Here's how the part is built. I have some questions about the finished solid (model axes, mm). A direction names the side the tool comes from. Round coordinates to 2 decimals unless told otherwise and drop trailing zeros. Write each loop counter-clockwise with the first axis right and the second up, starting at its lowest first coordinate (ties: lowest second). Pieces come first, ordered by that corner, then holes. Notation, with made-up numbers: (38.5, 38.5) -> (63.5, 38.5) arc R18 cw to (63.5, 48.5) -> close; hole circle Ø8 at (2.25, 36). An arc over 180 degrees is marked (long way). Answer in a Markdown table with one row per item.
from build123d import *

# Parameters (mm, degrees)
F0_R      = 50
F1_DEPTH  = 198
F1_TAPER  = -5
F1_FACE_R = 67.3227553781
F2_DEPTH  = 103
F2_TAPER  = 5
F3_DEPTH  = 25
F3_FACE_R = 58.311423035
F4_DEPTH  = 25
F4_TAPER  = -20
F5_R      = 45
F6_DEPTH  = 304


with BuildPart() as f1:
    # F0 (on Top) → F1 (new body)
    with BuildSketch(Plane.XY):
        Circle(F0_R)
    extrude(amount=F1_DEPTH, taper=F1_TAPER)

    # F1_face (on face) → F2 (join)
    with BuildSketch(Plane.XY.offset(198)):
        Circle(F1_FACE_R)
    extrude(amount=F2_DEPTH, taper=F2_TAPER)

    # F3 (add): a face of the model
    f3_faces = [f1.faces().sort_by_distance(p)[0] for p in [
        (0, 0, 301),
    ]]
    extrude(f3_faces, amount=F3_DEPTH)

    # F3_face (on face) → F4 (join)
    with BuildSketch(Plane.XY.offset(326)):
        Circle(F3_FACE_R)
    extrude(amount=F4_DEPTH, taper=F4_TAPER)

    # F5 (on face) → F6 (cut)
    with BuildSketch(Plane.XY.offset(351)):
        Circle(F5_R)
    extrude(amount=-F6_DEPTH, mode=Mode.SUBTRACT)


solid = f1.part
1) We'd pull the mould along Z, two halves only. Please class faces 4 (the face through (54, 22, 313)), 5 (the face through (-46.648, -35.768, 100.386)), 6 (the face through (14, -44, 351)): +Z half, -Z half, draft (parallel to the pull), parting line (faces both ways), or undercut.
Response:
| item | result |
|---|---|
| face 4 | undercut |
| face 5 | -Z half |
| face 6 | +Z half |
2) Which directions (+Z, -Z, +X, -X, +Y, -Y) give clear straight access to the entire face, cutting with the end or side of a thin tool? Please do faces 1 (the face through (-12.76, -57.48, 327.56)), 2 (the face through (-1, 1, 0)), 3 (the face through (-1, 1, 47)).
Response:
| item | result |
|---|---|
| face 1 | none |
| face 2 | -Z, +X, -X, +Y, -Y |
| face 3 | +Z |
3) I want a section at B-B, the plane z = 321.5. List the corners of the cut face in (x, y) for me.
Response:
| item | result |
|---|---|
| outline | circle Ø116.62 at (0, 0); hole circle Ø90 at (0, 0) |
4) For pin 1 (2 mm diameter, centred on y = -26.5, z = 179.5, fed in from +X); pin 2 (12 mm diameter, centred on x = -15, y = 23.5, fed in from +Z); pin 3 (8 mm diameter, centred on y = -26.5, z = 117, fed in from +X); pin 4 (6 mm diameter, centred on x = -39.5, y = -35, fed in from -Z), each with a flat end and sliding along its axis, tell me the tip position at first contact or that it passes through.
Response:
| item | result |
|---|---|
| pin 1 | stops at x = 60.56 |
| pin 2 | stops at z = 47 |
| pin 3 | stops at x = 55.92 |
| pin 4 | stops at z = 0 |
5) I want a section at C-C, the plane z = 231.5. List the corners of the cut face in (x, y) for me.
Response:
| item | result |
|---|---|
| outline | circle Ø128.78 at (0, 0); hole circle Ø90 at (0, 0) |
6) I want a section at A-A, the plane x = 0. List the corners of the cut face in (y, z) for me, and give its area (3 significant figures).
Response:
| item | result |
|---|---|
| outline | (-67.41, 351) -> (-58.31, 326) -> (-58.31, 301) -> (-67.32, 198) -> (-50, 0) -> (50, 0) -> (67.32, 198) -> (58.31, 301) -> (58.31, 326) -> (67.41, 351) -> (45, 351) -> (45, 47) -> (-45, 47) -> (-45, 351) -> close |
| area | 14,900 mm^2 |
7) I need wall thicknesses on line 1 (Z direction, x = 12, y = 34.5); line 2 (Y direction, x = 0, z = 287); line 3 (Y direction, x = -15.5, z = 313). Which ranges of each line are inside material? Lowest first, please. Write a range as [from, to].
Response:
| item | result |
|---|---|
| line 1 | z = [0, 47] |
| line 2 | y = [-59.54, -45], [45, 59.54] |
| line 3 | y = [-56.21, -42.25], [42.25, 56.21] |
